```python
from build123d import *

# Parameters (mm, degrees)
BOSS_EXTRUDE1_DEPTH = 16
SKETCH2_R           = 2.658036829
CUT_EXTRUDE1_DEPTH  = 16
SKETCH3_R           = 1.75
CUT_EXTRUDE2_DEPTH  = 5
CHAMFER1_SIZE       = 1


with BuildPart() as part:
    # Sketch1 → Boss-Extrude1 (new body)
    with BuildSketch(Plane.XY):
        Polygon((-8.547486034, 7.854748603), (11.452513966, 7.854748603), (11.452513966, -2.145251397), (-3.547486034, -2.145251397), (-3.547486034, -11.145251397), (-8.547486034, -11.145251397), align=None)
    extrude(amount=BOSS_EXTRUDE1_DEPTH)

    # Sketch2 → Cut-Extrude1 (cut)
    with BuildSketch(Plane(origin=(0, 7.854748603, 0), x_dir=(1, 0, 0), z_dir=(0, 1, 0))):
        with Locations((5.952513966, -8)):
            Circle(SKETCH2_R)
    extrude(amount=-CUT_EXTRUDE1_DEPTH, mode=Mode.SUBTRACT)

    # Sketch3 → Cut-Extrude2 (cut)
    with BuildSketch(Plane(origin=(-3.547486034, 0, 0), x_dir=(0, 0, -1), z_dir=(1, 0, 0))):
        with Locations((-12, -7.145251397)):
            Circle(SKETCH3_R)
        with Locations((-4, -7.145251397)):
            Circle(SKETCH3_R)
    extrude(amount=-CUT_EXTRUDE2_DEPTH, mode=Mode.SUBTRACT)

    # Chamfer1
    chamfer1_edges = [part.edges().sort_by_distance(p)[0] for p in [
        (11.452513966, 2.854748603, 16),
        (11.452513966, 2.854748603, 0),
    ]]
    chamfer(chamfer1_edges, length=CHAMFER1_SIZE)


solid = part.part
```
The model under review builds one solid part; all positions refer to its coordinate system, in mm. A direction names the side the tool comes from. Give positions to 0.01 mm unless a question says otherwise; leave off trailing zeros. Write each loop counter-clockwise with the first axis right and the second up, starting at its lowest first coordinate (ties: lowest second). Pieces come first, ordered by that corner, then holes. Notation, with made-up numbers: M 33.25,44 L 68.25,44 A35 ccw 68.25,83 Z; hole C 5.5,28.5 d9. An arc over 180 degrees is marked long. Write item = value, one per line. Start each with the question number.
Q1. Clearance check with flat-ended pins moving along their axes: pin 1 (7.5 mm diameter, centred on x = 7.5, z = 10, fed in from -Y); pin 2 (2 mm diameter, centred on x = -2.5, y = -8, fed in from +Z); pin 3 (6 mm diameter, centred on y = -5.5, z = 4, fed in from -X); pin 4 (2.5 mm diameter, centred on y = -7, z = 5.5, fed in from +X). State where each tip first meets the part, or that it passes through.
Q2. We need section B-B (y = -0.75). State the section outline as (x, z) points.
Q3. Mouldability with a two-part tool opening along Z and no side actions: class faces 3 (the face through (1, 7.855, 8)), 4 (the face through (5.4, 2.9, 10.6)), 5 (the face through (-6, -8.7, 11.2)), 6 (the face through (-1, 1, 16)) as released by +Z, released by -Z, zero draft, split by the parting line, or undercut.
Q4. We need section D-D (y = -6). State the section outline as (x, z) points.
Q5. Machinability: for faces 1 (the face through (2, -2.145, 8)), 2 (the face through (10.96, 2.92, 15.49)), which of the approach directions +Z, -Z, +X, -X, +Y, -Y give a long, thin tool a straight path to every point of the face, cutting with its end or side? Answer none if there is none.
Q6. We need section C-C (x = 4.5). State the section outline as (y, z) points.
Q7. We need section A-A (z = 12). State the section outline as (x, y) points.
Q8. For line 1 (Y direction, x = -5.1, z = 12); line 2 (X direction, y = 4.25, z = 8); line 3 (Y direction, x = 6.5, z = 1), list the stretches that pass through material, from the lowest coordinate up.
Result set:
q1.pin_1 = -2.15
q1.pin_2 = through
q1.pin_3 = -8.55
q1.pin_4 = -3.55
q2.outline = M -8.55,0 L 10.45,0 L 11.45,1 L 11.45,15 L 10.45,16 L -8.55,16 Z; hole C 5.95,8 d5.32
q3.face_3 = zero draft
q3.face_4 = undercut
q3.face_5 = undercut
q3.face_6 = released by +Z
q4.outline = M -8.55,0 L -3.55,0 L -3.55,2.68 L -8.55,2.68 Z; M -8.55,5.32 L -3.55,5.32 L -3.55,10.68 L -8.55,10.68 Z; M -8.55,13.32 L -3.55,13.32 L -3.55,16 L -8.55,16 Z
q5.face_1 = +Z, -Z, +X, -Y
q5.face_2 = +Z, +X, +Y, -Y
q6.outline = M -2.15,0 L 7.85,0 L 7.85,5.77 L -2.15,5.77 Z; M -2.15,10.23 L 7.85,10.23 L 7.85,16 L -2.15,16 Z
q7.outline = M -8.55,-11.15 L -3.55,-11.15 L -3.55,-8.9 L -8.55,-8.9 Z; M -8.55,-5.4 L -3.55,-5.4 L -3.55,-2.15 L 11.45,-2.15 L 11.45,7.85 L -8.55,7.85 Z
q8.line_1 = -11.15 to -8.9, -5.4 to 7.85
q8.line_2 = -8.55 to 3.29, 8.61 to 11.45
q8.line_3 = -2.15 to 7.85
